Verification items for the finished model (mm, model axes). A direction names the side the tool comes from. Round coordinates to 2 decimals unless told otherwise and drop trailing zeros. Order: outer loops, then holes, each group sorted by start corner. A loop starts at its lowest first (then second) coordinate and runs counter-clockwise, first axis right, second up. Notation, with made-up numbers: (22.5, 1.25) -> (26.5, 1.25) arc R25 cw to (26.5, 28.25) -> close; hole circle Ø9 at (-10.5, 81). An arc over 180 degrees is marked (long way). Answer in a Markdown table with one row per item. Add a question column.
```python
from build123d import *

# Parameters (mm, degrees)
F0_W     = 10
F0_H     = 10
F0_R     = 1.500154
F3_DEPTH = 1.5
F2_W     = 10
F2_H     = 10
F2_R     = 1.500154
F4_DEPTH = 1.5
F1_W     = 10
F1_H     = 10
F1_R     = 1.500154
F5_DEPTH = 1.5


with BuildPart() as f3:
    # F0 (on Front) → F3 (new body)
    with BuildSketch(Plane.XZ):
        with Locations((5, 5)):
            Rectangle(F0_W, F0_H)
        with Locations((5, 5)):
            Circle(F0_R, mode=Mode.SUBTRACT)
    extrude(amount=-F3_DEPTH)

    # F2 (on Top) → F4 (join)
    with BuildSketch(Plane.XY):
        with Locations((5, 5)):
            Rectangle(F2_W, F2_H)
        with Locations((5, 5)):
            Circle(F2_R, mode=Mode.SUBTRACT)
    extrude(amount=F4_DEPTH)

    # F1 (on Right) → F5 (join)
    with BuildSketch(Plane.YZ):
        with Locations((5, 5)):
            Rectangle(F1_W, F1_H)
        with Locations((5, 5)):
            Circle(F1_R, mode=Mode.SUBTRACT)
    extrude(amount=F5_DEPTH)


solid = f3.part
```
1) Draft check along X on faces 3 (the face through (3.89, 6.01, 0.74)), 4 (the face through (3, 1, 10)), 5 (the face through (1.5, 7, 6)), 6 (the face through (3.89, 0.74, 6.01)). Enter one of: +X half, -X half, draft (parallel to the pull), parting line (faces both ways), or undercut.
2) Thickness scan on L1, parallel to Y at x = 5, z = 0.55; L2, parallel to Y at x = 3, z = 5.5. Record the ranges inside material, lowest first. Write a range as [from, to].
3) Tool access check on faces 1 (the face through (0.74, 3.89, 6.01)), 2 (the face through (7, 6, 1.5)). Record the directions out of +Z, -Z, +X, -X, +Y, -Y that give a thin tool (end or side, any length) a straight path to the whole face; none if there is none.
4) Depth check by flat-ended pin: P1, Ø4, axis at x = 6.5, y = 7, coming from the +Z side; P2, Ø4, axis at x = 5, z = 5, coming from the +Y side; P3, Ø2.5, axis at y = 5, z = 5, coming from the -X side. Enter the tip coordinate at first touch or a pass-through.
5) Cross-section at C-C, the plane z = 0.75. Record the boundary of the cut face in (x, y), and give its area (3 significant figures).
6) Cross-section at D-D, the plane y = 6.75. Record the boundary of the cut face in (x, z).
7) Cross-section at A-A, the plane x = 5. Record the boundary of the cut face in (y, z).
Results below:
| question | item | result |
|---|---|---|
| 1 | face 3 | undercut |
| 1 | face 4 | draft |
| 1 | face 5 | +X half |
| 1 | face 6 | undercut |
| 2 | L1 | [0, 3.5], [6.5, 10] |
| 2 | L2 | [0, 1.5] |
| 3 | face 1 | +X, -X |
| 3 | face 2 | +Z, +X, +Y |
| 4 | P1 | z = 1.5 |
| 4 | P2 | y = 1.5 |
| 4 | P3 | through |
| 5 | outline | (0, 0) -> (10, 0) -> (10, 10) -> (0, 10) -> close; hole circle Ø3 at (5, 5) |
| 5 | area | 92.9 mm² |
| 6 | outline | (0, 0) -> (10, 0) -> (10, 1.5) -> (1.5, 1.5) -> (1.5, 10) -> (0, 10) -> close |
| 7 | outline | (0, 0) -> (3.5, 0) -> (3.5, 1.5) -> (1.5, 1.5) -> (1.5, 3.5) -> (0, 3.5) -> close; (0, 6.5) -> (1.5, 6.5) -> (1.5, 10) -> (0, 10) -> close; (6.5, 0) -> (10, 0) -> (10, 1.5) -> (6.5, 1.5) -> close |
